Geometry check sheet. Reference: the model listing, model coordinates, mm. Face numbers are marked on the shaded views. A direction names the side the tool comes from. Round coordinates to 2 decimals unless told otherwise and drop trailing zeros. Order: outer loops, then holes, each group sorted by start corner. A loop starts at its lowest first (then second) coordinate and runs counter-clockwise, first axis right, second up.
(1) Sectioned sample at A-A (z = -1.5). Give the number of separate pieces and of enclosed holes in the cut face, plus the area to 3 significant figures.
(2) Release check for a two-part mould opening along X. For the marked faces 1, 2 and 3 record: +X half, -X half, draft (parallel to the pull), parting line (faces both ways), or undercut.
(3) Sectioned sample at C-C (z = -15.5). Record the boundary of the cut face in (x, y) (3 decimals).
(4) Set-up check for the marked faces 4, 5, 6, 7 and 8: record each of +Z, -Z, +X, -X, +Y, -Y from which the full face is reachable in a straight line by a thin tool's end or side.
(5) Go/stop test with flat-tipped pins: pin 1 (1.6 mm diameter, centred on y = -4, z = -3, fed in from -X); pin 2 (5.5 mm diameter, centred on x = -2, z = -32.5, fed in from -Y); pin 3 (4 mm diameter, centred on x = -1, z = -33, fed in from +Y). Record where each tip stops, or that it passes through.
(6) Material ranges on line 1 along Y through (x, z) = (0, -5.5) (3 decimals); line 2 along Y through (x, z) = (0, -10.5) (3 decimals); line 3 along X through (y, z) = (-4.25, -3.5), recorded low to high.
(7) Sectioned sample at B-B (z = -10). Record the boundary of the cut face in (x, y) (3 decimals).
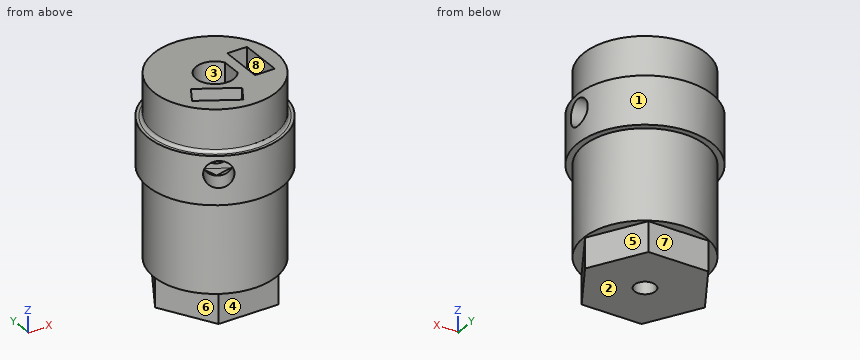
from build123d import *

# Parameters (mm, degrees)
SKETCH_2_R               = 1.75
EXTRUDE_1_DEPTH          = 5
SKETCH_3_W               = 2.5
SKETCH_3_H               = 7.4
EXTRUDE_2_DEPTH          = 15
CUT_EXTRUDE_1_DEPTH      = 0.2
CUT_EXTRUDE_1_DEPTH_BACK = 12
SKETCH_4_R               = 2.2
SKETCH_9_W               = 3.3
SKETCH_9_H               = 7.2
CUT_EXTRUDE_5_DEPTH      = 13
CUT_EXTRUDE_6_DEPTH      = 3.3
CUT_EXTRUDE_7_DEPTH      = 10
CUT_EXTRUDE_7_DEPTH_BACK = 5
SKETCH_12_R              = 2.2
CUT_EXTRUDE_8_DEPTH      = 3.4
FILLET_2_R               = 0.5


with BuildPart() as part:
    # Эскиз1 → Повернуть1 (revolve)
    with BuildSketch(Plane(origin=(0, 0, 0), x_dir=(0, 0, -1), z_dir=(1, 0, 0)), mode=Mode.PRIVATE) as revolve_1_sk:
        Polygon((0, 0), (0, 7.025), (7, 7.025), (7, 8.025), (15, 8.025), (15, 7.025), (30, 7.025), (30, -1.4), (14.5, -1.4), (14.5, 0), align=None)
    revolve(revolve_1_sk.sketch.rotate(Axis((0, -3.15, 0), (0, 0, -1)), 90), axis=Axis((0, -3.15, 0), (0, 0, -1)))

    # Эскиз2 → Бобышка-Вытянуть1 (add)
    with BuildSketch(Plane(origin=(0, 0, -30), x_dir=(-1, 0, 0), z_dir=(0, 0, -1))):
        Polygon((4.994079828, 5.5), (-4.994079828, 5.5), (-9.988159657, -3.15), (-4.994079828, -11.8), (4.994079828, -11.8), (9.988159657, -3.15), align=None)
        with Locations(Location((0, -3.15, 0), (0, 0, 180))):
            Circle(SKETCH_2_R, mode=Mode.SUBTRACT)
    extrude(amount=EXTRUDE_1_DEPTH)

    # Эскиз3 → Бобышка-Вытянуть2 (add)
    with BuildSketch(Plane.XY):
        with BuildLine():
            Line((2.7, -4.772498074), (2.7, -1.527501926))
            ThreePointArc((2.7, -1.527501926), (3.15, -3.15), (2.7, -4.772498074))
        make_face()
        with Locations((5.7, -3.15)):
            Rectangle(SKETCH_3_W, SKETCH_3_H)
    extrude(amount=-EXTRUDE_2_DEPTH)

    # Эскиз4 → Вырез-Вытянуть1 (cut, two sides: drawn at the far end of the back side and taken through both)
    with BuildSketch(Plane.ZY.offset(-2.7).offset(-CUT_EXTRUDE_1_DEPTH_BACK)):
        with Locations(Location((-10, -3.15, 0), (0, 0, 180))):
            Circle(SKETCH_4_R)
    extrude(amount=CUT_EXTRUDE_1_DEPTH + CUT_EXTRUDE_1_DEPTH_BACK, mode=Mode.SUBTRACT)

    # Скругление1: read off the stored shape, not the designer's step
    # Скругление1 outline → Скругление1 (revolve)
    with BuildSketch(Plane.XZ.offset(3.15)):
        with BuildLine():
            Line((3.15, -14.5), (3.15, -13.5))
            ThreePointArc((3.15, -13.5), (2.857106781, -14.207106781), (2.15, -14.5))
            Line((2.15, -14.5), (3.15, -14.5))
        make_face()
    revolve(axis=Axis((0, -3.15, 0), (0, 0, 1)))

    # Эскиз9 → Вырез-Вытянуть5 (cut)
    with BuildSketch(Plane.XY):
        with Locations((6, -3.15)):
            Rectangle(SKETCH_9_W, SKETCH_9_H)
        Polygon((-6.942691454, -7.975094339), (-5.292691454, -5.117210506), (0.942691454, -8.717210506), (-0.707308546, -11.575094339), align=None)
    extrude(amount=-CUT_EXTRUDE_5_DEPTH, mode=Mode.SUBTRACT)

    # Эскиз10 → Вырез-Вытянуть6 (cut)
    with BuildSketch(Plane(origin=(4.35, 0, 0), x_dir=(0, 0, -1), z_dir=(1, 0, 0))):
        Polygon((5.843078062, -3.15), (7.921539031, -6.75), (12.078460969, -6.75), (14.156921938, -3.15), (12.078460969, 0.45), (7.921539031, 0.45), align=None)
    extrude(amount=CUT_EXTRUDE_6_DEPTH, mode=Mode.SUBTRACT)

    # Эскиз12 → Вырез-Вытянуть7 (cut, two sides: drawn at the far end of the back side and taken through both)
    with BuildSketch(Plane(origin=(-3.538990011, -6.129710506, 0), x_dir=(0.8660254037844364, -0.500000000000004, 0), z_dir=(-0.500000000000004, -0.8660254037844365, 0)).offset(-CUT_EXTRUDE_7_DEPTH_BACK)):
        with Locations(Location((1.575, -10, 0), (0, 0, 180))):
            Circle(SKETCH_12_R)
    extrude(amount=CUT_EXTRUDE_7_DEPTH + CUT_EXTRUDE_7_DEPTH_BACK, mode=Mode.SUBTRACT)

    # Эскиз13 → Вырез-Вытянуть8 (cut)
    with BuildSketch(Plane(origin=(-3.538990011, -6.129710506, 0), x_dir=(0.8660254037844364, -0.500000000000004, 0), z_dir=(-0.500000000000004, -0.8660254037844365, 0))):
        Polygon((-2.025, -7.921539031), (-2.025, -12.078460969), (1.575, -14.156921938), (5.175, -12.078460969), (5.175, -7.921539031), (1.575, -5.843078062), align=None)
    extrude(amount=CUT_EXTRUDE_8_DEPTH, mode=Mode.SUBTRACT)

    # Скругление2
    fillet_2_edges = [part.edges().sort_by_distance(p)[0] for p in [
        (-10.175, -3.15, -7),
    ]]
    fillet(fillet_2_edges, radius=FILLET_2_R)


solid = part.part
Answer below:
1. separate pieces: 1
1. enclosed holes: 3
1. area: 248 mm2
2. face 1: parting line
2. face 2: draft
2. face 3: undercut
3. outline: circle Ø20.35 at (0, -3.15); hole circle Ø3.5 at (0, -3.15)
4. face 4: -Z, +X, -X, -Y
4. face 5: -Z, +X, +Y
4. face 6: -Z, -X, -Y
4. face 7: -Z, +X, -X, +Y
4. face 8: +Z
5. pin 1: stops at x = -10.17
5. pin 2: stops at y = -13.29
5. pin 3: stops at y = 5.5
6. line 1: y = -13.325 to -10.35, -8.173 to -6.3, 0 to 7.025
6. line 2: y = -14.325 to -10.35, -8.173 to -7.435, 0 to 8.025
6. line 3: x = -10.12 to -2.95, 2.7 to 4.35, 7.65 to 10.12
7. outline: (-7.383, -11.538) - (-5.78, -8.762) - (-6.993, -8.062) - (-5.293, -5.117) - (-4.08, -5.817) - (-3.032, -4.002) arc R3.15 cw to (2.5, -1.234) - (2.5, -0.95) - (4.35, -0.95) - (4.35, 0.45) - (7.65, 0.45) - (7.65, -0.95) - (10.956, -0.95) arc R11.175 ccw (long way) to start; (-3.573, -13.738) arc R11.175 ccw to (10.956, -5.35) - (7.65, -5.35) - (7.65, -6.75) - (4.35, -6.75) - (4.35, -5.35) - (2.5, -5.35) - (2.5, -5.066) arc R3.15 cw to (0.778, -6.202) - (-0.27, -8.017) - (0.943, -8.717) - (-0.757, -11.662) - (-1.97, -10.962) - close
